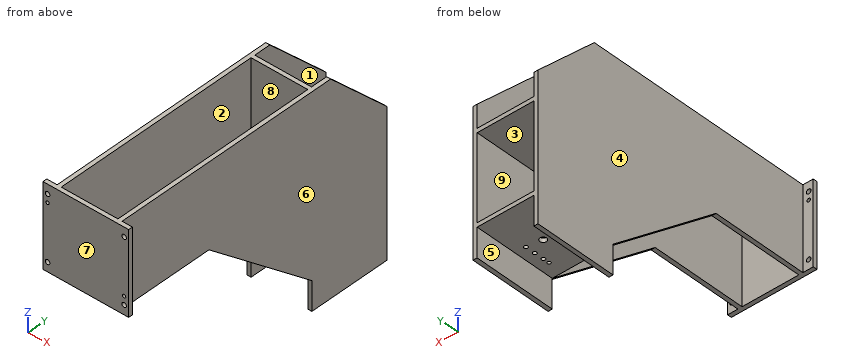
from build123d import *

# Parameters (mm, degrees)
BOSS_EXTRUDE1_DEPTH      = 10
BOSS_EXTRUDE1_DEPTH_BACK = 147
SKETCH3_W                = 137
SKETCH3_H                = 500
CUT_EXTRUDE1_DEPTH       = 705.5
SKETCH4_W                = 137
SKETCH4_H                = 200
BOSS_EXTRUDE2_DEPTH      = 10
CUT_EXTRUDE3_REACH       = 82
SKETCH6_R                = 4.5
SKETCH6_R_2              = 8
SKETCH6_R_3              = 4
SKETCH9_W                = 25
SKETCH9_H                = 200
BOSS_EXTRUDE4_DEPTH      = 10
SKETCH10_R               = 5.5
SKETCH10_R_2             = 4
CUT_EXTRUDE4_DEPTH       = 716.5
SKETCH11_W               = 137
SKETCH11_H               = 430
BOSS_EXTRUDE5_DEPTH      = 10
SKETCH12_W               = 10
SKETCH12_H               = 200
BOSS_EXTRUDE6_DEPTH      = 137


with BuildPart() as part:
    # Sketch1 → Boss-Extrude1 (new body, two sides)
    with BuildSketch(Plane(origin=(0, 0, 0), x_dir=(0, 0, -1), z_dir=(1, 0, 0))) as boss_extrude1_sk:
        Polygon((200, 515.5), (200, 241.396673703), (430, 515.5), align=None)
        Polygon((200, 0), (200, 515.5), (500, 515.5), (500, 715.5), (150, 715.5), (0, 565.5), (0, 0), align=None)
    extrude(amount=BOSS_EXTRUDE1_DEPTH)
    extrude(boss_extrude1_sk.sketch, amount=-BOSS_EXTRUDE1_DEPTH_BACK)

    # Sketch3 → Cut-Extrude1 (cut)
    with BuildSketch(Plane(origin=(0, 715.5, 0), x_dir=(1, 0, 0), z_dir=(0, 1, 0))):
        with Locations((-68.5, 250)):
            Rectangle(SKETCH3_W, SKETCH3_H)
    extrude(amount=-CUT_EXTRUDE1_DEPTH, mode=Mode.SUBTRACT)

    # Sketch4 → Boss-Extrude2 (add)
    with BuildSketch(Plane(origin=(0, 0, -430), x_dir=(-1, 0, 0), z_dir=(0, 0, -1))):
        with Locations((68.5, 615.5)):
            Rectangle(SKETCH4_W, SKETCH4_H)
    extrude(amount=-BOSS_EXTRUDE2_DEPTH)

    # Sketch6 → Cut-Extrude3 (cut, up to next)
    with BuildSketch(Plane.XY.offset(-420), mode=Mode.PRIVATE) as cut_extrude3_sk1:
        with Locations((-111, 567.7)):
            Circle(SKETCH6_R)
    cut_extrude3_tool1 = extrude(cut_extrude3_sk1.sketch, amount=-CUT_EXTRUDE3_REACH, mode=Mode.PRIVATE) & part.part
    add(cut_extrude3_tool1.solids().sort_by_distance((-111, 567.7, -420))[0], mode=Mode.SUBTRACT)
    # Sketch6 → Cut-Extrude3 (cut, up to next)
    with BuildSketch(Plane.XY.offset(-420), mode=Mode.PRIVATE) as cut_extrude3_sk2:
        with Locations((-26, 567.7)):
            Circle(SKETCH6_R)
    cut_extrude3_tool2 = extrude(cut_extrude3_sk2.sketch, amount=-CUT_EXTRUDE3_REACH, mode=Mode.PRIVATE) & part.part
    add(cut_extrude3_tool2.solids().sort_by_distance((-26, 567.7, -420))[0], mode=Mode.SUBTRACT)
    # Sketch6 → Cut-Extrude3 (cut, up to next)
    with BuildSketch(Plane.XY.offset(-420), mode=Mode.PRIVATE) as cut_extrude3_sk3:
        with Locations((-111, 614.2)):
            Circle(SKETCH6_R)
    cut_extrude3_tool3 = extrude(cut_extrude3_sk3.sketch, amount=-CUT_EXTRUDE3_REACH, mode=Mode.PRIVATE) & part.part
    add(cut_extrude3_tool3.solids().sort_by_distance((-111, 614.2, -420))[0], mode=Mode.SUBTRACT)
    # Sketch6 → Cut-Extrude3 (cut, up to next)
    with BuildSketch(Plane.XY.offset(-420), mode=Mode.PRIVATE) as cut_extrude3_sk4:
        with Locations((-26, 614.2)):
            Circle(SKETCH6_R)
    cut_extrude3_tool4 = extrude(cut_extrude3_sk4.sketch, amount=-CUT_EXTRUDE3_REACH, mode=Mode.PRIVATE) & part.part
    add(cut_extrude3_tool4.solids().sort_by_distance((-26, 614.2, -420))[0], mode=Mode.SUBTRACT)
    # Sketch6 → Cut-Extrude3 (cut, up to next)
    with BuildSketch(Plane.XY.offset(-420), mode=Mode.PRIVATE) as cut_extrude3_sk5:
        with Locations((-63, 609)):
            Circle(SKETCH6_R_2)
    cut_extrude3_tool5 = extrude(cut_extrude3_sk5.sketch, amount=-CUT_EXTRUDE3_REACH, mode=Mode.PRIVATE) & part.part
    add(cut_extrude3_tool5.solids().sort_by_distance((-63, 609, -420))[0], mode=Mode.SUBTRACT)
    # Sketch6 → Cut-Extrude3 (cut, up to next)
    with BuildSketch(Plane.XY.offset(-420), mode=Mode.PRIVATE) as cut_extrude3_sk6:
        with Locations((-111, 629.2)):
            Circle(SKETCH6_R_3)
    cut_extrude3_tool6 = extrude(cut_extrude3_sk6.sketch, amount=-CUT_EXTRUDE3_REACH, mode=Mode.PRIVATE) & part.part
    add(cut_extrude3_tool6.solids().sort_by_distance((-111, 629.2, -420))[0], mode=Mode.SUBTRACT)
    # Sketch6 → Cut-Extrude3 (cut, up to next)
    with BuildSketch(Plane.XY.offset(-420), mode=Mode.PRIVATE) as cut_extrude3_sk7:
        with Locations((-26, 552.7)):
            Circle(SKETCH6_R_3)
    cut_extrude3_tool7 = extrude(cut_extrude3_sk7.sketch, amount=-CUT_EXTRUDE3_REACH, mode=Mode.PRIVATE) & part.part
    add(cut_extrude3_tool7.solids().sort_by_distance((-26, 552.7, -420))[0], mode=Mode.SUBTRACT)
    # Sketch6 → Cut-Extrude3 (cut, up to next)
    with BuildSketch(Plane.XY.offset(-420), mode=Mode.PRIVATE) as cut_extrude3_sk8:
        with Locations((-111, 590.7)):
            Circle(SKETCH6_R)
    cut_extrude3_tool8 = extrude(cut_extrude3_sk8.sketch, amount=-CUT_EXTRUDE3_REACH, mode=Mode.PRIVATE) & part.part
    add(cut_extrude3_tool8.solids().sort_by_distance((-111, 590.7, -420))[0], mode=Mode.SUBTRACT)
    # Sketch6 → Cut-Extrude3 (cut, up to next)
    with BuildSketch(Plane.XY.offset(-420), mode=Mode.PRIVATE) as cut_extrude3_sk9:
        with Locations((-26, 590.7)):
            Circle(SKETCH6_R)
    cut_extrude3_tool9 = extrude(cut_extrude3_sk9.sketch, amount=-CUT_EXTRUDE3_REACH, mode=Mode.PRIVATE) & part.part
    add(cut_extrude3_tool9.solids().sort_by_distance((-26, 590.7, -420))[0], mode=Mode.SUBTRACT)

    # Sketch9 → Boss-Extrude4 (add)
    with BuildSketch(Plane.XZ):
        with Locations((-159.5, -100)):
            Rectangle(SKETCH9_W, SKETCH9_H)
        with Locations((22.5, -100)):
            Rectangle(SKETCH9_W, SKETCH9_H)
    extrude(amount=-BOSS_EXTRUDE4_DEPTH)

    # Sketch10 → Cut-Extrude4 (cut, through all)
    with BuildSketch(Plane.XZ):
        with Locations((-161, -22.5)):
            Circle(SKETCH10_R)
        with Locations((24, -22.5)):
            Circle(SKETCH10_R)
        with Locations((24, -177.5)):
            Circle(SKETCH10_R)
        with Locations((-161, -177.5)):
            Circle(SKETCH10_R)
        with Locations((-161, -42.5)):
            Circle(SKETCH10_R_2)
        with Locations((24, -157.5)):
            Circle(SKETCH10_R_2)
    extrude(amount=-CUT_EXTRUDE4_DEPTH, mode=Mode.SUBTRACT)

    # Sketch11 → Boss-Extrude5 (add)
    with BuildSketch(Plane.XZ.offset(-515.5)):
        with Locations((-68.5, -215)):
            Rectangle(SKETCH11_W, SKETCH11_H)
    extrude(amount=-BOSS_EXTRUDE5_DEPTH)

    # Sketch12 → Boss-Extrude6 (add)
    with BuildSketch(Plane(origin=(-137, 0, 0), x_dir=(0, 0, -1), z_dir=(1, 0, 0))):
        with Locations((210, 615.5)):
            Rectangle(SKETCH12_W, SKETCH12_H)
    extrude(amount=BOSS_EXTRUDE6_DEPTH)


solid = part.part
Input: part model. Units: mm. Frame: model coordinates. Face numbers are marked on the shaded views. A direction names the side the tool comes from. Coordinates: 2 decimals unless noted, no trailing zeros. Order: outer loops, then holes, each group sorted by start corner. A loop starts at its lowest first (then second) coordinate and runs counter-clockwise, first axis right, second up. Notation, with made-up numbers: M 46.5,-20.5 L 97.5,-20.5 A10 ccw 97.5,-7.5 Z; hole C 68,33.25 d3. An arc over 180 degrees is marked long. Answer in a Markdown table with one row per item.
(1) Access query for the marked faces 1, 2, 3, 4 and 5. Directions: +Z, -Z, +X, -X, +Y, -Y. A direction counts if a zero-diameter tool reaches every point of the face in a straight line with its end or side. Return the directions, or none.
Numbers:
| item | result |
|---|---|
| face 1 | +Z, +Y |
| face 2 | +Z, -Z |
| face 3 | +Y |
| face 4 | +Z, -Z, -X, +Y |
| face 5 | -Z, +Y, -Y |
(2) Section query B-B, the plane y = 143.5. Output: boundary loops of the cut face in (x, z).
Numbers:
| item | result |
|---|---|
| outline | M -147,-200 L -137,-200 L -137,0 L -147,0 Z; M 0,-200 L 10,-200 L 10,0 L 0,0 Z |
(3) Section query C-C, the plane z = -273.5. Output: boundary loops of the cut face in (x, y), plus the area to 3 significant figures.
Numbers:
| item | result |
|---|---|
| outline | M -147,328.99 L -137,328.99 L -137,515.5 L 0,515.5 L 0,328.99 L 10,328.99 L 10,715.5 L 0,715.5 L 0,525.5 L -137,525.5 L -137,715.5 L -147,715.5 Z |
| area | 9,100 mm^2 |
(4) Material intervals for line 1 (Y direction, x = -111, z = -422); line 2 (X direction, y = 590, z = -424); line 3 (X direction, y = 590.7, z = -426.75), sorted ascending. Write a range as [from, to].
Numbers:
| item | result |
|---|---|
| line 1 | y = [515.5, 563.2], [572.2, 586.2], [595.2, 609.7], [618.7, 625.2], [633.2, 715.5] |
| line 2 | x = [-147, -115.45], [-106.55, -30.45], [-21.55, 10] |
| line 3 | x = [-147, -115.5], [-106.5, -30.5], [-21.5, 10] |
(5) Section query D-D, the plane y = 314. Output: boundary loops of the cut face in (x, z), plus the area to 3 significant figures.
Numbers:
| item | result |
|---|---|
| outline | M -147,-260.92 L -137,-260.92 L -137,0 L -147,0 Z; M 0,-260.92 L 10,-260.92 L 10,0 L 0,0 Z |
| area | 5,220 mm^2 |
(6) Contact query for flat-ended pins moving along their axis: pin 1 Ø11.5 at (x, y) = (-26, 614.2) entering from -Z; pin 2 Ø1.5 at (y, z) = (82.5, -144) entering from -X; pin 3 Ø12.5 at (x, z) = (28.5, -140.5) entering from +Y. Output: stop coordinate, or through.
Numbers:
| item | result |
|---|---|
| pin 1 | stops at z = -430 |
| pin 2 | stops at x = -147 |
| pin 3 | stops at y = 10 |
(7) Section query A-A, the plane x = -93.5. Output: boundary loops of the cut face in (y, z), plus the area to 3 significant figures.
Numbers:
| item | result |
|---|---|
| outline | M 0,-200 L 10,-200 L 10,0 L 0,0 Z; M 515.5,-430 L 715.5,-430 L 715.5,-420 L 525.5,-420 L 525.5,-215 L 715.5,-215 L 715.5,-205 L 525.5,-205 L 525.5,0 L 515.5,0 Z |
| area | 10,100 mm^2 |
(8) Draft query along X for the marked faces 6, 7, 8 and 9. Return one class per face: pulls with the +X half, pulls with the -X half, needs draft (parallel to the pull), parting line crosses it, or undercut.
Numbers:
| item | result |
|---|---|
| face 6 | pulls with the +X half |
| face 7 | needs draft |
| face 8 | undercut |
| face 9 | undercut |
